```python
from build123d import *

# Parameters (mm, degrees)
SKETCH1_W           = 20
SKETCH1_H           = 10
BOSS_EXTRUDE1_DEPTH = 5
SKETCH2_W           = 8
SKETCH2_H           = 10
BOSS_EXTRUDE2_DEPTH = 50
CUT_EXTRUDE1_DEPTH  = 10
BOSS_EXTRUDE3_START = 5
BOSS_EXTRUDE3_DEPTH = 5
CUT_EXTRUDE2_DEPTH  = 2.5


with BuildPart() as part:
    # Sketch1 → Boss-Extrude1 (new body)
    with BuildSketch(Plane.XY):
        Rectangle(SKETCH1_W, SKETCH1_H)
    extrude(amount=BOSS_EXTRUDE1_DEPTH)

    # Sketch2 → Boss-Extrude2 (add)
    with BuildSketch(Plane.XY.offset(5)):
        Rectangle(SKETCH2_W, SKETCH2_H)
    extrude(amount=BOSS_EXTRUDE2_DEPTH)

    # Sketch3 → Cut-Extrude1 (cut)
    with BuildSketch(Plane.XY.offset(5)):
        with BuildLine():
            Line((-7.5, 1.7), (-10, 1.7))
            Line((-10, 1.7), (-10, -1.7))
            Line((-10, -1.7), (-7.5, -1.7))
            ThreePointArc((-7.5, -1.7), (-5.8, 0), (-7.5, 1.7))
        make_face()
        with BuildLine():
            Line((7.5, 1.7), (10, 1.7))
            Line((10, 1.7), (10, -1.7))
            Line((10, -1.7), (7.5, -1.7))
            ThreePointArc((7.5, -1.7), (5.8, 0), (7.5, 1.7))
        make_face()
    extrude(amount=-CUT_EXTRUDE1_DEPTH, mode=Mode.SUBTRACT)

    # Sketch4 → Boss-Extrude3 (add)
    with BuildSketch(Plane.XY.offset(55).offset(BOSS_EXTRUDE3_START)):
        with BuildLine():
            Line((-7.5, 1.7), (-10, 1.7))
            Line((-10, 1.7), (-10, 5))
            Line((-10, 5), (10, 5))
            Line((10, 5), (10, 1.7))
            Line((10, 1.7), (7.5, 1.7))
            ThreePointArc((7.5, 1.7), (5.8, 0), (7.5, -1.7))
            Line((7.5, -1.7), (10, -1.7))
            Line((10, -1.7), (10, -5))
            Line((10, -5), (-10, -5))
            Line((-10, -5), (-10, -1.7))
            Line((-10, -1.7), (-7.5, -1.7))
            ThreePointArc((-7.5, -1.7), (-5.8, 0), (-7.5, 1.7))
        make_face()
    extrude(amount=-BOSS_EXTRUDE3_DEPTH)

    # Sketch5 → Cut-Extrude2 (cut)
    with BuildSketch(Plane.XY.offset(5)):
        Polygon((-4.75, 1.58771324), (-4.75, -1.58771324), (-7.5, -3.175426481), (-10.25, -1.58771324), (-10.25, 1.58771324), (-7.5, 3.175426481), align=None)
    cut_extrude2 = extrude(amount=-CUT_EXTRUDE2_DEPTH, mode=Mode.SUBTRACT)

    # Mirror1: Cut-Extrude2 across plane
    add(cut_extrude2.mirror(Plane(origin=(0, 0, 0), x_dir=(0, 0, 1), z_dir=(1, 0, 0))), mode=Mode.SUBTRACT)


solid = part.part
```
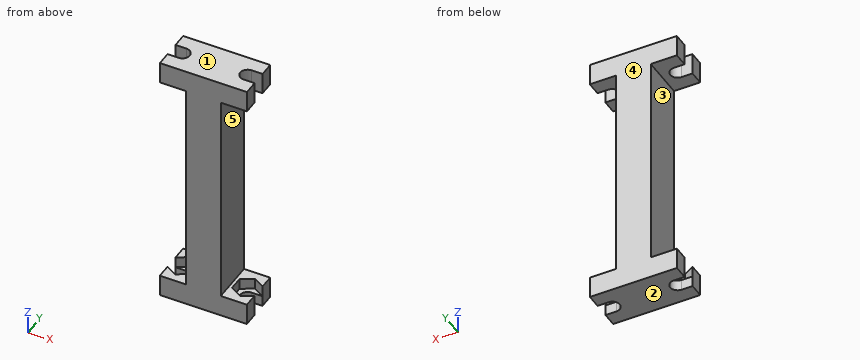
The listing builds one solid part. Answer for the finished solid, in the listing's coordinates (mm). Face numbers are marked on the shaded views. A direction names the side the tool comes from. Coordinates: 2 decimals unless noted, no trailing zeros. Write each loop counter-clockwise with the first axis right and the second up, starting at its lowest first coordinate (ties: lowest second). Pieces come first, ordered by that corner, then holes. Notation, with made-up numbers: M -35,-5.75 L -19,-5.75 A28 cw -19,27.25 Z; hole C 81,41 d11. An arc over 180 degrees is marked long. Use a Markdown table: item, result. Add a question column.
1. Section A-A (x = -6.75) is taken. Give the vertices of the cut face in (y, z).
2. Section D-D (y = -2.25) is taken. Give the vertices of the cut face in (x, z).
3. Section B-B (y = 0) is taken. Give the vertices of the cut face in (x, z), plus the area to 3 significant figures.
4. For a pull along Z with two mould halves and no side action, classify the marked faces 1, 2 and 3 as +Z half, -Z half, draft (parallel to the pull), parting line (faces both ways), or undercut.
5. Section C-C (z = 32) is taken. Give the vertices of the cut face in (x, y), plus the area to 3 significant figures.
6. Straight lines are drawn through the part: line 1 along Z through (x, y) = (-5.25, -1); line 2 along Z through (x, y) = (6.75, 3.25); line 3 along X through (y, z) = (4.5, 40.5). For each, find the intervals that lie inside material, in ascending order. Write a range as [from, to].
7. Which of the six approach directions +Z, -Z, +X, -X, +Y, -Y give full straight-line access (tool end or side, diameter ignored) to the marked faces 4 and 5?
8. Given P1, Ø3, axis at y = -3.5, z = 20.5, coming from the +X side; P2, Ø2, axis at x = -1.5, y = -3.5, coming from the -Z side; P3, Ø0.8, axis at y = 0, z = 4.5, coming from the -X side; P4, Ø1.5, axis at y = 2, z = 7, coming from the -X side, each flat-ended and moving along its own axis, determine where each tip first touches the part or whether it passes through.
Data:
| question | item | result |
|---|---|---|
| 1 | outline | M -5,0 L -1.53,0 L -1.53,2.5 L -2.74,2.5 L -2.74,5 L -5,5 Z; M -5,55 L -1.53,55 L -1.53,60 L -5,60 Z; M 1.53,0 L 5,0 L 5,5 L 2.74,5 L 2.74,2.5 L 1.53,2.5 Z; M 1.53,55 L 5,55 L 5,60 L 1.53,60 Z |
| 2 | outline | M -10,0 L 10,0 L 10,5 L 9.1,5 L 9.1,2.5 L 5.9,2.5 L 5.9,5 L 4,5 L 4,55 L 10,55 L 10,60 L -10,60 L -10,55 L -4,55 L -4,5 L -5.9,5 L -5.9,2.5 L -9.1,2.5 L -9.1,5 L -10,5 Z |
| 3 | outline | M -5.8,0 L 5.8,0 L 5.8,2.5 L 4.75,2.5 L 4.75,5 L 4,5 L 4,55 L 5.8,55 L 5.8,60 L -5.8,60 L -5.8,55 L -4,55 L -4,5 L -4.75,5 L -4.75,2.5 L -5.8,2.5 Z |
| 3 | area | 511 mm2 |
| 4 | face 1 | +Z half |
| 4 | face 2 | -Z half |
| 4 | face 3 | undercut |
| 5 | outline | M -4,-5 L 4,-5 L 4,5 L -4,5 Z |
| 5 | area | 80.0 mm2 |
| 6 | line 1 | z = [0, 2.5], [55, 60] |
| 6 | line 2 | z = [0, 5], [55, 60] |
| 6 | line 3 | x = [-4, 4] |
| 7 | face 4 | +Z, -Z, +X, -X, +Y |
| 7 | face 5 | +X, +Y, -Y |
| 8 | P1 | stops at x = 4 |
| 8 | P2 | stops at z = 0 |
| 8 | P3 | stops at x = -4.75 |
| 8 | P4 | stops at x = -4 |
